For this review, take the finished solid that the model builds, in its own axes (mm). Face numbers are marked on the shaded views. A direction names the side the tool comes from. Give positions to 0.01 mm unless a question says otherwise; leave off trailing zeros. Order: outer loops, then holes, each group sorted by start corner. A loop starts at its lowest first (then second) coordinate and runs counter-clockwise, first axis right, second up. Notation, with made-up numbers: (30.25, 71) - (45.25, 71) arc R28 cw to (45.25, 91) - close; hole circle Ø6 at (36, 77.25). An arc over 180 degrees is marked (long way). Use a Markdown table: item, result. Add a question column.
1) Wall thickness on L1, parallel to Z at x = -37.5, y = 40; L2, parallel to Y at x = 81, z = -34.5; L3, parallel to Z at x = -34, y = -61: over which ranges is each line inside the solid? List them lowest first.
2) We need section C-C on x = 10. Write out the cut boundary in (y, z), then the cut area to 3 significant figures.
3) Mouldability with a two-part tool opening along Y and no side actions: class the marked faces 4, 5 and 6 as released by +Y, released by -Y, zero draft, split by the parting line, or undercut.
4) We need section A-A on z = -23. Write out the cut boundary in (x, y), then the cut area to 3 significant figures.
5) We need section B-B on x = 65. Write out the cut boundary in (y, z).
6) Clearance check with flat-ended pins moving along their axes: P1, Ø4, axis at x = 63.5, y = 48, coming from the +Z side; P2, Ø12, axis at y = -100, z = 27, coming from the +X side; P3, Ø15, axis at y = -144.5, z = -36, coming from the +X side. State where each tip first meets the part, or that it passes through.
7) We need section D-D on x = -68.5. Write out the cut boundary in (y, z).
8) Machinability: for the marked faces 1, 2 and 3, which of the approach directions +Z, -Z, +X, -X, +Y, -Y give a long, thin tool a straight path to every point of the face, cutting with its end or side? Answer none if there is none.
```python
from build123d import *

# Parameters (mm, degrees)
F0_W          = 235.2761279326
F0_H          = 107.4857413769
F1_DEPTH      = 151.892
F1_DEPTH_BACK = 76.2
F3_DEPTH      = 237.236
F3_DEPTH_BACK = 76.2
F4_W          = 77.9956504703
F4_H          = 36.5806035697
F5_DEPTH      = 158.242
F6_R          = 15.4248239937
F6_R_2        = 15.9308513278
F6_R_3        = 15.1256103557
F6_R_4        = 15.251280461
F7_DEPTH      = 184.658
F7_DEPTH_BACK = 146.812
F8_W          = 88.170285026
F8_H          = 30.4754237933
F9_DEPTH      = 160.528
F10_W         = 82.4058901053
F10_H         = 30.2224318786
F11_DEPTH     = 127.762


with BuildPart() as f1:
    # F0 (on Front) → F1 (new body, two sides)
    with BuildSketch(Plane.XZ) as f1_sk:
        with Locations((1.289183856, 0)):
            Rectangle(F0_W, F0_H)
    extrude(amount=F1_DEPTH)
    extrude(f1_sk.sketch, amount=-F1_DEPTH_BACK)

    # F2 (on Front) → F3 (cut, two sides)
    with BuildSketch(Plane.XZ) as f3_sk:
        Polygon((126.138061285, 57.2444498539), (-31.619194895, 57.2444498539), (126.138061285, -59.499990195), align=None)
    extrude(amount=F3_DEPTH, mode=Mode.SUBTRACT)
    extrude(f3_sk.sketch, amount=-F3_DEPTH_BACK, mode=Mode.SUBTRACT)

    # F4 (on Right) → F5 (cut)
    with BuildSketch(Plane.YZ):
        with Locations((-0.1611486077, 52.5342617184)):
            Rectangle(F4_W, F4_H)
    extrude(amount=-F5_DEPTH, mode=Mode.SUBTRACT)

    # F6 (on Right) → F7 (cut, two sides)
    with BuildSketch(Plane.YZ) as f7_sk:
        with Locations((-46.7329323292, 13.6170089245)):
            Circle(F6_R)
        with Locations((-46.7329323292, -29.7318119556)):
            Circle(F6_R_2)
        with Locations((39.4812710583, -29.7318119556)):
            Circle(F6_R_3)
        with Locations((39.4812710583, 15.550785698)):
            Circle(F6_R_4)
    extrude(amount=-F7_DEPTH, mode=Mode.SUBTRACT)
    extrude(f7_sk.sketch, amount=F7_DEPTH_BACK, mode=Mode.SUBTRACT)

    # F8 (on face) → F9 (cut)
    with BuildSketch(Plane(origin=(0, 0, -53.7428706884), x_dir=(1, 0, 0), z_dir=(0, 0, -1))):
        with Locations((74.2732988048, 136.6542881033)):
            Rectangle(F8_W, F8_H)
    extrude(amount=-F9_DEPTH, mode=Mode.SUBTRACT)

    # F10 (on face) → F11 (cut)
    with BuildSketch(Plane(origin=(0, 0, -53.7428706884), x_dir=(1, 0, 0), z_dir=(0, 0, -1))):
        with Locations((-75.1459350577, 136.7807840607)):
            Rectangle(F10_W, F10_H)
    extrude(amount=-F11_DEPTH, mode=Mode.SUBTRACT)


solid = f1.part
```
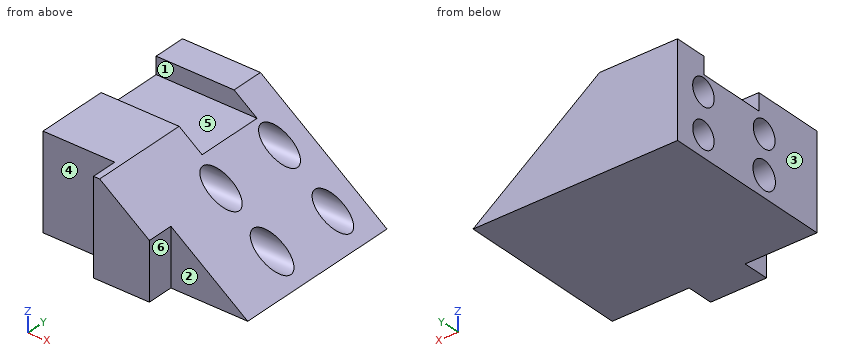
Checked values:
| question | item | result |
|---|---|---|
| 1 | L1 | -53.74 to -44.85, -14.62 to 0.31, 30.79 to 53.74 |
| 1 | L2 | -121.42 to -61.93, -31.53 to 25.13, 53.84 to 76.2 |
| 1 | L3 | -53.74 to -36.82, -22.64 to 7.75, 19.48 to 53.74 |
| 2 | outline | (-151.89, -53.74) - (76.2, -53.74) - (76.2, 26.45) - (50.15, 26.45) arc R15.25 cw (long way) to (28.81, 26.45) - (-38.17, 26.45) arc R15.42 cw (long way) to (-55.3, 26.45) - (-151.89, 26.45) - close; hole circle Ø31.86 at (-46.73, -29.73); hole circle Ø30.25 at (39.48, -29.73) |
| 2 | area | 15,400 mm² |
| 3 | face 4 | released by -Y |
| 3 | face 5 | undercut |
| 3 | face 6 | zero draft |
| 4 | outline | (-116.35, -121.67) - (-33.94, -121.67) - (-33.94, -151.89) - (30.19, -151.89) - (30.19, -121.42) - (76.82, -121.42) - (76.82, -61.17) - (-116.35, -61.17) - close; (-116.35, -32.29) - (76.82, -32.29) - (76.82, 25.94) - (-116.35, 25.94) - close; (-116.35, 53.03) - (76.82, 53.03) - (76.82, 76.2) - (-116.35, 76.2) - close |
| 4 | area | 29,300 mm² |
| 5 | outline | (-121.42, -53.74) - (76.2, -53.74) - (76.2, -14.26) - (-42.95, -14.26) arc R15.93 cw (long way) to (-50.51, -14.26) - (-121.42, -14.26) - close; hole circle Ø30.25 at (39.48, -29.73) |
| 6 | P1 | z = -11.67 |
| 6 | P2 | x = 17.36 |
| 6 | P3 | x = 30.19 |
| 7 | outline | (-121.67, -53.74) - (76.2, -53.74) - (76.2, 53.74) - (38.84, 53.74) - (38.84, 34.24) - (-39.16, 34.24) - (-39.16, 53.74) - (-121.67, 53.74) - close; hole circle Ø31.86 at (-46.73, -29.73); hole circle Ø30.85 at (-46.73, 13.62); hole circle Ø30.5 at (39.48, 15.55); hole circle Ø30.25 at (39.48, -29.73) |
| 8 | face 1 | +Z, +X, -X |
| 8 | face 2 | +Z, -Z, +X, -Y |
| 8 | face 3 | +Z, -Z, -X, +Y, -Y |
